Input: part model. Units: mm. Frame: model coordinates. Give positions to 0.01 mm unless a question says otherwise; leave off trailing zeros. Loops run counter-clockwise (first coordinate to the right, second up) from the corner with the lowest first, then second, coordinate; pieces in that order, holes last. Notation, with made-up numbers: (48, -21) - (76, -21) arc R8 ccw to (76, -15) - close; hole circle Ø11 at (6, 41.25). An arc over 180 degrees is marked (long way). Answer as a JSON object with one key per item and string values.
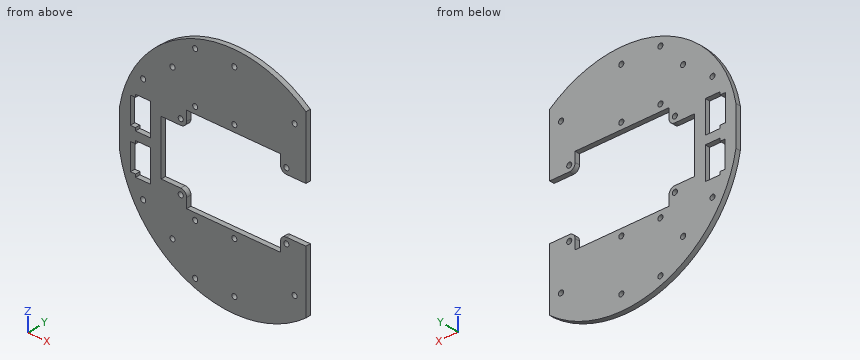
from build123d import *

# Parameters (mm, degrees)
SKETCH1_R           = 1.651
BOSS_EXTRUDE1_DEPTH = 3.175
CUT_EXTRUDE1_START  = -3.175
CUT_EXTRUDE1_DEPTH  = 3.175


with BuildPart() as part:
    # Sketch1 → Boss-Extrude1 (new body)
    with BuildSketch(Plane(origin=(0, 0, 0), x_dir=(1, 0, 0), z_dir=(0, 1, 0))):
        with BuildLine():
            Line((-73.916912814, 12.7), (-73.916912814, -12.7))
            ThreePointArc((-73.916912814, -12.7), (75, 0), (-73.916912814, 12.7))
        make_face()
        with Locations(Location((-34.29, 21.59, 0), (0, 0, 270))):
            Circle(SKETCH1_R, mode=Mode.SUBTRACT)
        with Locations(Location((34.29, 21.59, 0), (0, 0, 270))):
            Circle(SKETCH1_R, mode=Mode.SUBTRACT)
        with Locations(Location((-34.29, -21.59, 0), (0, 0, 270))):
            Circle(SKETCH1_R, mode=Mode.SUBTRACT)
        with Locations(Location((34.29, -21.59, 0), (0, 0, 270))):
            Circle(SKETCH1_R, mode=Mode.SUBTRACT)
        with Locations(Location((39.626912814, -48.698461806, 0), (0, 0, 270))):
            Circle(SKETCH1_R, mode=Mode.SUBTRACT)
        with Locations(Location((-58.676912814, -34.29, 0), (0, 0, 270))):
            Circle(SKETCH1_R, mode=Mode.SUBTRACT)
        with Locations(Location((-58.676912814, 34.29, 0), (0, 0, 270))):
            Circle(SKETCH1_R, mode=Mode.SUBTRACT)
        with Locations(Location((39.626912814, 48.698461806, 0), (0, 0, 270))):
            Circle(SKETCH1_R, mode=Mode.SUBTRACT)
        with Locations(Location((0.498087186, -65.123461806, 0), (0, 0, 90))):
            Circle(SKETCH1_R, mode=Mode.SUBTRACT)
        with Locations(Location((0.498087186, -32.273461806, 0), (0, 0, 90))):
            Circle(SKETCH1_R, mode=Mode.SUBTRACT)
        with Locations(Location((0.498087186, 32.273461806, 0), (0, 0, 270))):
            Circle(SKETCH1_R, mode=Mode.SUBTRACT)
        with Locations(Location((0.498087186, 65.123461806, 0), (0, 0, 270))):
            Circle(SKETCH1_R, mode=Mode.SUBTRACT)
        with Locations(Location((-39.626912814, -48.698461806, 0), (0, 0, 270))):
            Circle(SKETCH1_R, mode=Mode.SUBTRACT)
        with Locations(Location((-24.901912814, -32.273461806, 0), (0, 0, 270))):
            Circle(SKETCH1_R, mode=Mode.SUBTRACT)
        with Locations(Location((-24.901912814, -65.123461806, 0), (0, 0, 270))):
            Circle(SKETCH1_R, mode=Mode.SUBTRACT)
        with Locations(Location((-24.901912814, 65.123461806, 0), (0, 0, 90))):
            Circle(SKETCH1_R, mode=Mode.SUBTRACT)
        with Locations(Location((-39.626912814, 48.698461806, 0), (0, 0, 90))):
            Circle(SKETCH1_R, mode=Mode.SUBTRACT)
        with Locations(Location((-24.901912814, 32.273461806, 0), (0, 0, 90))):
            Circle(SKETCH1_R, mode=Mode.SUBTRACT)
        with BuildLine():
            Line((-30.48, 27.94), (30.48, 27.94))
            Line((30.48, 27.94), (30.48, 21.59))
            ThreePointArc((30.48, 21.59), (31.595923164, 18.895923164), (34.29, 17.78))
            Line((34.29, 17.78), (46.99, 17.78))
            Line((46.99, 17.78), (46.99, -17.78))
            Line((46.99, -17.78), (34.29, -17.78))
            ThreePointArc((34.29, -17.78), (31.595923164, -18.895923164), (30.48, -21.59))
            Line((30.48, -21.59), (30.48, -27.94))
            Line((30.48, -27.94), (-30.48, -27.94))
            Line((-30.48, -27.94), (-30.48, -21.59))
            ThreePointArc((-30.48, -21.59), (-31.595923164, -18.895923164), (-34.29, -17.78))
            Line((-34.29, -17.78), (-46.99, -17.78))
            Line((-46.99, -17.78), (-46.99, 17.78))
            Line((-46.99, 17.78), (-34.29, 17.78))
            ThreePointArc((-34.29, 17.78), (-31.595923164, 18.895923164), (-30.48, 21.59))
            Line((-30.48, 21.59), (-30.48, 27.94))
        make_face(mode=Mode.SUBTRACT)
        Polygon((-66.997078327, -4.560855709), (-63.695078327, -4.560855709), (-63.695078327, -2.72123678), (-54.039956407, -2.72123678), (-54.039956407, -4.558974638), (-54.039956407, -21.70773678), (-54.039956407, -23.545474638), (-63.695078327, -23.545474638), (-63.695078327, -21.705855709), (-66.997078327, -21.705855709), align=None, mode=Mode.SUBTRACT)
        Polygon((-66.866956407, 21.70773678), (-63.564956407, 21.70773678), (-63.564956407, 23.54923678), (-54.039956407, 23.54923678), (-54.039956407, 21.70773678), (-54.039956407, 4.56273678), (-54.039956407, 2.72123678), (-63.564956407, 2.72123678), (-63.564956407, 4.56273678), (-66.866956407, 4.56273678), align=None, mode=Mode.SUBTRACT)
    extrude(amount=BOSS_EXTRUDE1_DEPTH)

    # Sketch2 → Cut-Extrude1 (cut)
    with BuildSketch(Plane(origin=(0, 3.175, 0), x_dir=(1, 0, 0), z_dir=(0, 1, 0)).offset(CUT_EXTRUDE1_START)):
        with BuildLine():
            Line((46.99, 58.454596911), (46.99, -58.454596911))
            ThreePointArc((46.99, -58.454596911), (75, 0), (46.99, 58.454596911))
        make_face()
    extrude(amount=CUT_EXTRUDE1_DEPTH, mode=Mode.SUBTRACT)


solid = part.part
Item 1: Cut plane A-A (x = 26). Return loops of the section in (y, z) (3 decimals), then the cut area to 3 significant figures.
Geometry check:
{"outline": "(0, -70.349) - (3.175, -70.349) - (3.175, -27.94) - (0, -27.94) - close; (0, 27.94) - (3.175, 27.94) - (3.175, 70.349) - (0, 70.349) - close", "area": "269 mm2"}
Item 2: Material intervals for line 1 (X direction, y = 1.5, z = -9.5); line 2 (X direction, y = 1.8, z = 3.5); line 3 (X direction, y = 0.8, z = -21.59), sorted ascending. Write a range as [from, to].
Geometry check:
{"line 1": "x = [-73.92, -66.87], [-54.04, -46.99]", "line 2": "x = [-73.92, -63.7], [-54.04, -46.99]", "line 3": "x = [-71.83, -66.87], [-54.04, -35.94], [-32.64, -30.48], [30.48, 32.64], [35.94, 46.99]"}
Item 3: Cut plane B-B (z = -14.5). Return loops of the section in (x, y) (3 decimals).
Geometry check:
{"outline": "(-73.585, 0) - (-66.867, 0) - (-66.867, 3.175) - (-73.585, 3.175) - close; (-54.04, 0) - (-46.99, 0) - (-46.99, 3.175) - (-54.04, 3.175) - close"}
Item 4: Cut plane C-C (y = 1.3). Give the number of separate pieces and of enclosed holes in the cut face, then the cut area to 3 significant figures.
Geometry check:
{"separate pieces": "1", "enclosed holes": "20", "area": "10,100 mm2"}
Item 5: Contact query for flat-ended pins moving along their axis: P1, Ø1.5, axis at y = 2, z = -25, coming from the -X side; P2, Ø1, axis at y = 2, z = 4, coming from the +X side; P3, Ø1, axis at x = -65, y = 2, coming from the +Z side. Output: stop coordinate, or through.
Geometry check:
{"P1": "stops at x = -70.97", "P2": "stops at x = -46.99", "P3": "stops at z = 38.27"}
